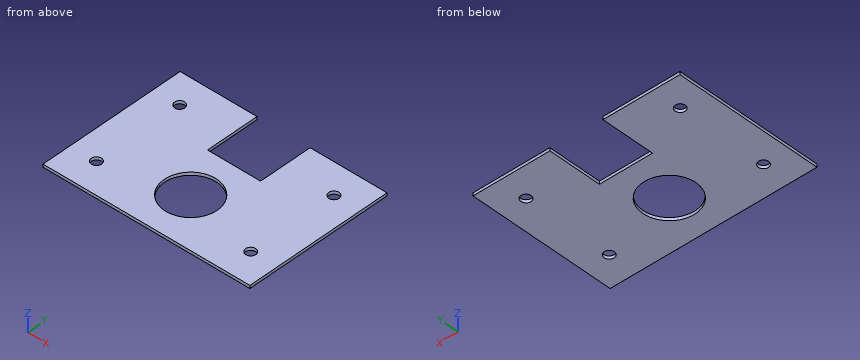
Autodesk Inventor part; units mm, degrees
ref_plane "YZ Plane" through (0, 0, 0) normal (1, 0, 0) x (0, 1, 0)
ref_plane "XZ Plane" through (0, 0, 0) normal (0, 1, 0) x (-1, 0, 0)
ref_plane "XY Plane" through (0, 0, 0) normal (0, 0, 1) x (1, 0, 0)
sketch "Sketch1" plane through (0, 0, 0) normal (0, 0, 1) x (1, 0, 0)
  line L0 (0, -55.6514) -> (0, 55.6514)
  line L1 (55.88, 39.751) -> (55.88, -39.751)
  line L2 (55.88, -39.751) -> (-55.88, -39.751)
  line L3 (-55.88, -39.751) -> (-55.88, 39.751)
  line L4 (-78.232, 0) -> (78.232, 0)
  line L5 (-14.351, 39.751) -> (-14.351, 11.049)
  line L6 (-14.351, 11.049) -> (14.351, 11.049)
  line L7 (14.351, 11.049) -> (14.351, 39.751)
  line L8 (-55.88, 39.751) -> (-14.351, 39.751)
  line L9 (14.351, 39.751) -> (55.88, 39.751)
  line L10 (0, -39.751) -> (0, -14.097)
  circle A0 centre (0, -14.097) radius 14.2875
  point P0 (0, 0)
  dimension "d0" = 111.76
  dimension "d1" = 79.502
  dimension "d2" = 28.702
  dimension "d3" = 28.702
  dimension "d4" = 25.654
  dimension "d5" = 28.575
extrude "Extrusion1" add sketch "Sketch1" along normal blind 1.5875 contours L2 L3 L4 A0 L0 | L0 A0 L4 L1 L2 | L4 L3 L8 L5 L6 L0 A0 | L4 A0 L0 L6 L7 L9 L1
sketch "Sketch2" plane through (0, 0, 1.5875) normal (0, 0, 1) x (1, 0, 0)
  line L0 (55.88, -39.751) -> (55.88, 39.751)
  line L1 (-55.88, -39.751) -> (55.88, -39.751)
  point P0 (0, 0)
  point P1 (41.656, 24.257)
  point P2 (41.656, -24.003)
  dimension "d15" = 48.26
  dimension "d16" = 14.224
  dimension "d17" = 14.224
  dimension "d18" = 15.748
hole "Hole1" at (41.656, 24.257, 1.5875) at (41.656, -24.003, 1.5875) direction (0, 0, -1) diameter 5.5118 end through all
mirror "Mirror1" about plane through (0, 0, 0) normal (1, 0, 0) of "Hole1"
properties part number "DIFF_PLATE_ROD_H"
Read the model definition and answer for the solid it produces. Units are mm, in the model's axes. Round coordinates to 2 decimals unless told otherwise and drop trailing zeros. Write each loop counter-clockwise with the first axis right and the second up, starting at its lowest first coordinate (ties: lowest second). Pieces come first, ordered by that corner, then holes.
Q1. Find section C-C on y = -2.5. Determine the outline of the cut face in (x, z).
Values:
outline: (-55.88, 0) - (-8.35, 0) - (-8.35, 1.59) - (-55.88, 1.59) - close; (8.35, 0) - (55.88, 0) - (55.88, 1.59) - (8.35, 1.59) - close
Q2. Find section B-B on z = 0.9. Determine the outline of the cut face in (x, y) (1 decimal), and give its area (3 significant figures).
Values:
outline: (-55.9, -39.8) - (55.9, -39.8) - (55.9, 39.8) - (14.4, 39.8) - (14.4, 11) - (-14.4, 11) - (-14.4, 39.8) - (-55.9, 39.8) - close; hole circle Ø5.5 at (-41.7, -24); hole circle Ø5.5 at (-41.7, 24.3); hole circle Ø28.6 at (0, -14.1); hole circle Ø5.5 at (41.7, -24); hole circle Ø5.5 at (41.7, 24.3)
area: 7,320 mm2
Q3. Find section D-D on y = -23.5. Determine the outline of the cut face in (x, z), and give its area (3 significant figures).
Values:
outline: (-55.88, 0) - (-44.37, 0) - (-44.37, 1.59) - (-55.88, 1.59) - close; (-38.95, 0) - (-10.76, 0) - (-10.76, 1.59) - (-38.95, 1.59) - close; (10.76, 0) - (38.95, 0) - (38.95, 1.59) - (10.76, 1.59) - close; (44.37, 0) - (55.88, 0) - (55.88, 1.59) - (44.37, 1.59) - close
area: 126 mm2
Q4. Flat-ended cylindrical pins translate along their axes: P1, Ø3.5, axis at x = 41.656, y = -24.003, coming from the +Z side; P2, Ø6.5, axis at x = -41.656, y = 24.257, coming from the +Z side. Find the tip coordinate at first contact, or state that the pin passes through.
Values:
P1: passes through
P2: stops at z = 1.59
Q5. Straight lines are drawn through the part: line 1 (X direction, y = -14, z = 1.3); line 2 (X direction, y = 29, z = 0.75); line 3 (X direction, y = -22, z = 0.75). For each, find the intervals that lie inside material, in ascending order.
Values:
line 1: x = -55.88 to -14.29, 14.29 to 55.88
line 2: x = -55.88 to -14.35, 14.35 to 55.88
line 3: x = -55.88 to -43.55, -39.76 to -11.9, 11.9 to 39.76, 43.55 to 55.88
Q6. Find section A-A on x = 0. Determine the outline of the cut face in (y, z), and give its area (3 significant figures).
Values:
outline: (-39.75, 0) - (-28.38, 0) - (-28.38, 1.59) - (-39.75, 1.59) - close; (0.19, 0) - (11.05, 0) - (11.05, 1.59) - (0.19, 1.59) - close
area: 35.3 mm2
